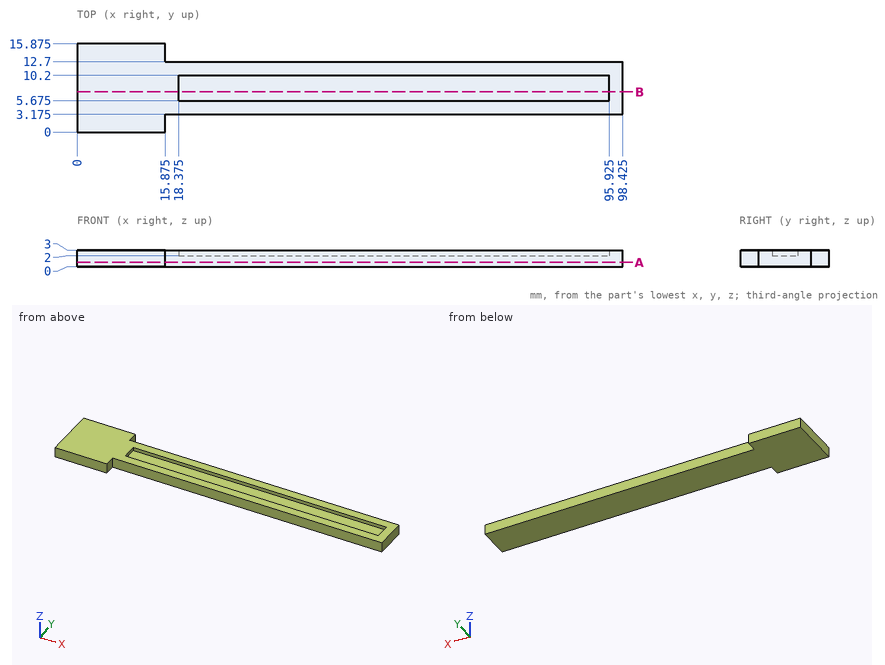
Here's the drawing with two shaded views (mm, measured from the low corner). I have some questions. Coordinates: 2 decimals unless noted, no trailing zeros. Loops run counter-clockwise (first coordinate to the right, second up) from the corner with the lowest first, then second, coordinate; pieces in that order, holes last. Notation, with made-up numbers: M 16.5,4.25 L 40.5,4.25 A22 ccw 40.5,36.25 Z; hole C -37.5,84 d4. An arc over 180 degrees is marked long. Put each result on its own line as item: value. Start each with the question number.
(1) I need wall thicknesses on probe 1 along X at (y, z) = (6.5, 2.75) (3 decimals); probe 2 along Y at (x, z) = (23, 2.45) (3 decimals); probe 3 along Y at (x, z) = (40.5, 1.95) (3 decimals). Which ranges of each line are inside material? Lowest first, please.
(2) Imagine slicing it at A-A on z = 0.8. List the corners of the cut face in (x, y) for me (3 decimals).
(3) Will these pins go through, and if not, where does the flat tip stop? pin 1 Ø1.1 at (x, z) = (46, 2.5) entering from -Y (3 decimals); pin 2 Ø1.1 at (x, z) = (59.5, 2.5) entering from +Y.
(4) Imagine slicing it at B-B on y = 7.25. List the corners of the cut face in (x, z) for me (3 decimals), and give its area (3 significant figures).
Worked answers:
1. probe 1: x = 0 to 18.375, 95.925 to 98.425
1. probe 2: y = 3.175 to 5.675, 10.2 to 12.7
1. probe 3: y = 3.175 to 12.7
2. outline: M 0,0 L 15.875,0 L 15.875,3.175 L 98.425,3.175 L 98.425,12.7 L 15.875,12.7 L 15.875,15.875 L 0,15.875 Z
3. pin 1: stops at y = 3.175
3. pin 2: stops at y = 12.7
4. outline: M 0,0 L 98.425,0 L 98.425,3 L 95.925,3 L 95.925,2 L 18.375,2 L 18.375,3 L 0,3 Z
4. area: 218 mm2
